Study the drawing (mm; zero at the part's minimum x, y, z) and answer. A direction names the side the tool comes from. Give positions to 0.01 mm unless a question says otherwise; leave off trailing zeros. Write each loop counter-clockwise with the first axis right and the second up, starting at its lowest first coordinate (ties: lowest second). Pieces come first, ordered by that corner, then holes.
1) Find section C-C (x = 40). Determine the outline of the cut face in (y, z) (1 decimal).
2) Find section A-A (x = 8). Determine the outline of the cut face in (y, z) (1 decimal).
3) Determine the mould class of the marked faces 1, 2, 3 and 4 for opening direction Y: pulls with the +Y half, pulls with the -Y half, needs draft (parallel to the pull), parting line crosses it, or undercut.
4) Find section D-D (y = 45). Determine the outline of the cut face in (x, z), plus the area to 3 significant figures.
5) Straight lines are drawn through the part: probe 1 along Y at (x, z) = (3, 5.45) (1 decimal); probe 2 along Y at (x, z) = (3.5, 3.85) (1 decimal); probe 3 along Y at (x, z) = (38, 4) (1 decimal). For each, find the intervals that lie inside material, in ascending order.
6) Given pin 1 Ø2 at (x, z) = (39.5, 2) entering from +Y (3 decimals); pin 2 Ø3 at (x, z) = (11.5, 4.5) entering from -Y; pin 3 Ø3 at (x, z) = (3.5, 3) entering from +Y (3 decimals), each flat-ended and moving along its own axis, determine where each tip first touches the part or whether it passes through.
7) A tool of negligible diameter and unlimited length cuts with its end or side. For the marked faces 5, 6, 7 and 8, from which of +Z, -Z, +X, -X, +Y, -Y can it reach the whole face along a straight path? Write none if from no direction.
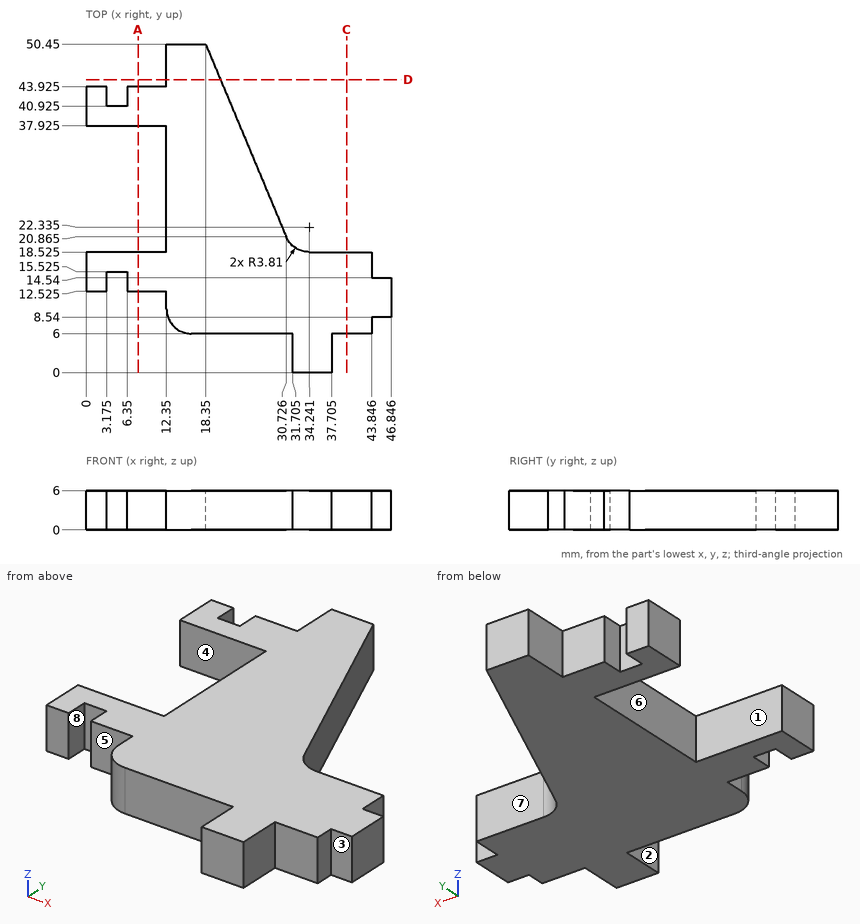
Results:
1. outline: (6, 0) - (18.5, 0) - (18.5, 6) - (6, 6) - close
2. outline: (12.5, 0) - (18.5, 0) - (18.5, 6) - (12.5, 6) - close; (37.9, 0) - (43.9, 0) - (43.9, 6) - (37.9, 6) - close
3. face 1: undercut
3. face 2: needs draft
3. face 3: pulls with the -Y half
3. face 4: undercut
4. outline: (12.35, 0) - (20.63, 0) - (20.63, 6) - (12.35, 6) - close
4. area: 49.7 mm2
5. probe 1: y = 12.5 to 18.5, 37.9 to 43.9
5. probe 2: y = 15.5 to 18.5, 37.9 to 40.9
5. probe 3: y = 6 to 18.5
6. pin 1: stops at y = 18.525
6. pin 2: stops at y = 7.68
6. pin 3: stops at y = 43.925
7. face 5: +Z, -Z, -X, -Y
7. face 6: +Z, -Z, -X
7. face 7: +Z, -Z, +X, +Y
7. face 8: +Z, -Z, -Y
